For this review, take the finished solid that the model builds, in its own axes (mm). A direction names the side the tool comes from. Coordinates: 2 decimals unless noted, no trailing zeros. Loops run counter-clockwise (first coordinate to the right, second up) from the corner with the lowest first, then second, coordinate; pieces in that order, holes last. Notation, with made-up numbers: (6.25, -37.75) -> (30.25, -37.75) arc R30 ccw to (30.25, 1.25) -> close; hole circle Ø3 at (63.5, 83). An arc over 180 degrees is marked (long way). Answer in a Markdown table with one row per item.
from build123d import *

# Parameters (mm, degrees)
BOSS_EXTRUDE1_DEPTH = 4
SKETCH4_W           = 26
SKETCH4_H           = 14
BOSS_EXTRUDE2_DEPTH = 3
FILLET1_R           = 1
FILLET3_R           = 3
FILLET4_R           = 3
SKETCH5_W           = 19.6
SKETCH5_H           = 7
BOSS_EXTRUDE3_DEPTH = 3
SKETCH8_W           = 19.6
SKETCH8_H           = 3
BOSS_EXTRUDE5_DEPTH = 5
SKETCH9_W           = 19.6
SKETCH9_H           = 3
BOSS_EXTRUDE6_DEPTH = 13
FILLET5_R           = 2


# Some blends are built 0.0001 mm under size
with BuildPart() as part:
    # Sketch1 → Boss-Extrude1 (new body)
    with BuildSketch(Plane(origin=(0, 0, 0), x_dir=(-1, 0, 0), z_dir=(0, 0, -1))):
        with BuildLine():
            Line((27.500000074, -16.263075607), (27.500000074, 0))
            Line((27.500000074, 0), (-20.499999926, 0))
            Line((-20.499999926, 0), (-20.499999926, -15.701236215))
            ThreePointArc((-20.499999926, -15.701236215), (3.511255672, -15.020548898), (27.500000074, -16.263075607))
        make_face()
    extrude(amount=-BOSS_EXTRUDE1_DEPTH)

    # Sketch4 → Boss-Extrude2 (add)
    with BuildSketch(Plane.XY.offset(4)):
        with Locations((-3.500000074, -7)):
            Rectangle(SKETCH4_W, SKETCH4_H)
    extrude(amount=BOSS_EXTRUDE2_DEPTH)

    # Fillet1
    fillet1_edges = [part.edges().sort_by_distance(p)[0] for p in [
        (20.499999926, 0, 2),
        (-27.500000074, 0, 2),
        (20.499999926, -15.701236215, 2),
        (-27.500000074, -16.263075607, 2),
    ]]
    fillet(fillet1_edges, radius=FILLET1_R)

    # Fillet3
    fillet3_edges = [part.edges().sort_by_distance(p)[0] for p in [
        (-3.500000074, -14, 7),
        (-16.500000074, -7, 7),
        (9.499999926, -7, 7),
    ]]
    fillet(fillet3_edges, radius=FILLET3_R - 0.0001)  # a hair under: the kernel refuses the full size

    # Fillet4
    # the kernel refuses this fillet: 3 mm, written as the material it takes off along each edge
    with BuildSketch(Plane(origin=(-13.500000074, -11, 7), x_dir=(-1, 0, 0), z_dir=(0, 1, 0))) as fillet4_piece_1:
        with BuildLine():
            CenterArc((0.0001, -2.9999), 2.9999, 0, 90)
            Line((3, -2.9999), (3, 0))
            Line((3, 0), (0.0001, 0))
        make_face()
    revolve(axis=Axis((-13.500000074, -11, 7), (0, 0, 1)), revolution_arc=90, mode=Mode.SUBTRACT)
    with BuildSketch(Plane(origin=(6.499999926, -11, 7), x_dir=(0, -1, 0), z_dir=(-1, 0, 0))) as fillet4_piece_2:
        with BuildLine():
            CenterArc((0.0001, -2.9999), 2.9999, 0, 90)
            Line((3, -2.9999), (3, 0))
            Line((3, 0), (0.0001, 0))
        make_face()
    revolve(axis=Axis((6.499999926, -11, 7), (0, 0, 1)), revolution_arc=90, mode=Mode.SUBTRACT)
    with BuildSketch(Plane(origin=(9.499999926, -14, 4), x_dir=(0, 1, 0), z_dir=(0, 0, 1))) as fillet4_piece_3:
        with BuildLine():
            CenterArc((FILLET4_R, FILLET4_R), FILLET4_R, 180, 90)
            Line((0, FILLET4_R), (0, 0))
            Line((0, 0), (FILLET4_R, 0))
        make_face()
    extrude(amount=3, mode=Mode.SUBTRACT)
    with BuildSketch(Plane(origin=(-16.500000074, -14, 4), x_dir=(0, 1, 0), z_dir=(0, 0, 1))) as fillet4_piece_4:
        with BuildLine():
            CenterArc((FILLET4_R, -FILLET4_R), FILLET4_R, 90, 90)
            Line((0, -FILLET4_R), (0, 0))
            Line((0, 0), (FILLET4_R, 0))
        make_face()
    extrude(amount=3, mode=Mode.SUBTRACT)

    # Sketch5 → Boss-Extrude3 (add)
    with BuildSketch(Plane(origin=(0, 0, 0), x_dir=(1, 0, 0), z_dir=(0, 1, 0))):
        with Locations((-3.500000074, -3.5)):
            Rectangle(SKETCH5_W, SKETCH5_H)
    extrude(amount=BOSS_EXTRUDE3_DEPTH)

    # Sketch8 → Boss-Extrude5 (add)
    with BuildSketch(Plane.XY.offset(7)):
        with Locations((-3.500000074, 1.5)):
            Rectangle(SKETCH8_W, SKETCH8_H)
    extrude(amount=BOSS_EXTRUDE5_DEPTH)

    # Sketch9 → Boss-Extrude6 (add)
    with BuildSketch(Plane.XZ):
        with Locations((-3.500000074, 13.5)):
            Rectangle(SKETCH9_W, SKETCH9_H)
    extrude(amount=-BOSS_EXTRUDE6_DEPTH)

    # Fillet5
    fillet5_edges = [part.edges().sort_by_distance(p)[0] for p in [
        (-3.500000074, 0, 15),
        (-3.500000074, 3, 0),
        (-3.500000074, 0, 7),
    ]]
    fillet(fillet5_edges, radius=FILLET5_R)


solid = part.part
Item 1: For L1, parallel to Z at x = -20.5, y = -14.25; L2, parallel to Z at x = 5, y = -10; L3, parallel to Y at x = -18, z = 1.5, list the stretches that pass through material, from the lowest coordinate up.
Worked answers:
| item | result |
|---|---|
| L1 | 0 to 4 |
| L2 | 0 to 7 |
| L3 | -15.54 to 0 |
Item 2: Insertion check: pin 1 (5.5 mm diameter, centred on x = 0, y = -3.5, fed in from +Z); pin 2 (8 mm diameter, centred on x = -1.5, z = 7, fed in from +Y); pin 3 (6 mm diameter, centred on y = 5, z = 2.5, fed in from -X). Each pin has a flat end and moves straight along its axis. Give the tip position at first contact, or say it passes through.
Worked answers:
| item | result |
|---|---|
| pin 1 | z = 7.44 |
| pin 2 | y = 3 |
| pin 3 | x = -13.3 |
Item 3: For faces 1 (the flat face through (13, 0, 3)), 2 (the flat face through (20.5, -8, 2)), 3 (the flat face through (-4, 0, 11)), 4 (the flat face through (-20, 0, 3)), 5 (the cylindrical face through (-3.36, 2.43, 0.6)), list the 3-axis set-ups (+Z, -Z, +X, -X, +Y, -Y) from which the entire face can be reached by the end or side of a thin tool; tool diameter is ignored.
Worked answers:
| item | result |
|---|---|
| face 1 | +Z, -Z, +X, +Y |
| face 2 | +Z, -Z, +X, +Y, -Y |
| face 3 | +Z, +X, -X, -Y |
| face 4 | +Z, -Z, -X, +Y |
| face 5 | -Z, +X, -X, +Y |
Item 4: The part is to be moulded in two halves that separate along Y. For faces 6 (the flat face through (-3, -7, 0)), 7 (the cylindrical face through (-3.36, -13.14, 6.1)), 8 (the flat face through (-4, 3, 7)), say which applies: +Y half, -Y half, draft (parallel to the pull), parting line (faces both ways), or undercut.
Worked answers:
| item | result |
|---|---|
| face 6 | draft |
| face 7 | -Y half |
| face 8 | +Y half |
Item 5: Take a section at D-D, the plane z = 3.5. State the section outline as (x, y) points.
Worked answers:
| item | result |
|---|---|
| outline | (-27.5, -15.17) arc R1 ccw to (-26.41, -16.16) arc R300 cw to (19.44, -15.63) arc R1 ccw to (20.5, -14.63) -> (20.5, -1) arc R1 ccw to (19.5, 0) -> (6.3, 0) -> (6.3, 3) -> (-13.3, 3) -> (-13.3, 0) -> (-26.5, 0) arc R1 ccw to (-27.5, -1) -> close |
Item 6: Take a section at B-B, the plane z = 1. State the section outline as (x, y) points, and give its area (3 significant figures).
Worked answers:
| item | result |
|---|---|
| outline | (-27.5, -15.17) arc R1 ccw to (-26.41, -16.16) arc R300 cw to (19.44, -15.63) arc R1 ccw to (20.5, -14.63) -> (20.5, -1) arc R1 ccw to (19.5, 0) -> (6.3, 0) -> (6.3, 2.73) -> (-13.3, 2.73) -> (-13.3, 0) -> (-26.5, 0) arc R1 ccw to (-27.5, -1) -> close |
| area | 789 mm² |
